Verification items for the finished model (mm, model axes). Face numbers are marked on the shaded views. A direction names the side the tool comes from. Give positions to 0.01 mm unless a question says otherwise; leave off trailing zeros. Order: outer loops, then holes, each group sorted by start corner. A loop starts at its lowest first (then second) coordinate and runs counter-clockwise, first axis right, second up. Notation, with made-up numbers: (63.5, 11.25) - (104.5, 11.25) arc R14 ccw to (104.5, 38.25) - close; hole circle Ø1 at (-17.5, 76). An arc over 180 degrees is marked (long way). Answer as a JSON object with one key per item and string values.
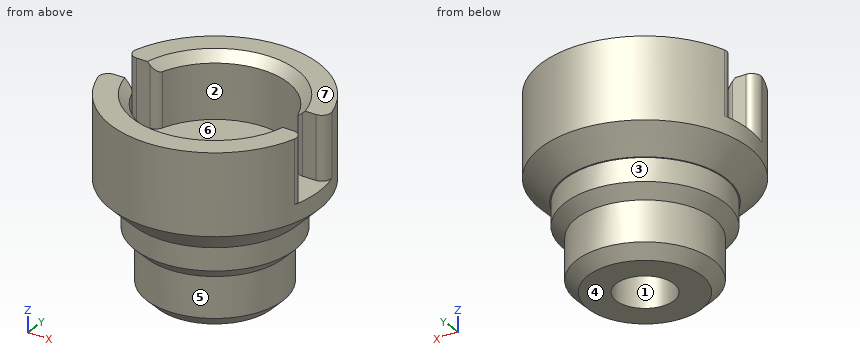
```python
from build123d import *

# Parameters (mm, degrees)
SKETCH1_R           = 2.95
SKETCH1_R_2         = 1.25
BOSS_EXTRUDE1_DEPTH = 3.75
SKETCH2_R           = 4.5
SKETCH2_R_2         = 1.25
BOSS_EXTRUDE2_DEPTH = 4.5
SKETCH3_R           = 3.15
CUT_EXTRUDE1_DEPTH  = 2.75
CHAMFER1_SIZE       = 0.4
CHAMFER2_SIZE       = 0.5
BOSS_EXTRUDE3_START = 1.5
SKETCH4_R           = 3.45
SKETCH4_R_2         = 1.25
BOSS_EXTRUDE3_DEPTH = 1.5
CHAMFER3_SIZE       = 1
CHAMFER6_SIZE       = 0.5
CUT_EXTRUDE2_REACH  = 12.419
SKETCH5_W           = 12.167806538
SKETCH5_H           = 1.5
FILLET1_R           = 0.4


with BuildPart() as part:
    # Sketch1 → Boss-Extrude1 (new body)
    with BuildSketch(Plane.XY):
        Circle(SKETCH1_R)
        Circle(SKETCH1_R_2, mode=Mode.SUBTRACT)
    extrude(amount=BOSS_EXTRUDE1_DEPTH)

    # Sketch2 → Boss-Extrude2 (add)
    with BuildSketch(Plane.XY.offset(3.75)):
        Circle(SKETCH2_R)
        Circle(SKETCH2_R_2, mode=Mode.SUBTRACT)
    extrude(amount=BOSS_EXTRUDE2_DEPTH)

    # Sketch3 → Cut-Extrude1 (cut)
    with BuildSketch(Plane.XY.offset(8.25)):
        Circle(SKETCH3_R)
    extrude(amount=-CUT_EXTRUDE1_DEPTH, mode=Mode.SUBTRACT)

    # Chamfer1
    chamfer1_edges = [part.edges().sort_by_distance(p)[0] for p in [
        (-3.15, 0, 8.25),
    ]]
    chamfer(chamfer1_edges, length=CHAMFER1_SIZE)

    # Chamfer2
    chamfer2_edges = [part.edges().sort_by_distance(p)[0] for p in [
        (-2.95, 0, 0),
    ]]
    chamfer(chamfer2_edges, length=CHAMFER2_SIZE)

    # Sketch4 → Boss-Extrude3 (add)
    with BuildSketch(Plane(origin=(0, 0, 3.75), x_dir=(-1, 0, 0), z_dir=(0, 0, -1)).offset(BOSS_EXTRUDE3_START)):
        with Locations(Location((0, 0, 0), (0, 0, 180))):
            Circle(SKETCH4_R)
        with Locations(Location((0, 0, 0), (0, 0, 180))):
            Circle(SKETCH4_R_2, mode=Mode.SUBTRACT)
    extrude(amount=-BOSS_EXTRUDE3_DEPTH)

    # Chamfer3
    chamfer3_edges = [part.edges().sort_by_distance(p)[0] for p in [
        (-4.5, 0, 3.75),
    ]]
    chamfer(chamfer3_edges, length=CHAMFER3_SIZE)

    # Chamfer6
    chamfer6_edges = [part.edges().sort_by_distance(p)[0] for p in [
        (-3.45, 0, 2.25),
    ]]
    chamfer(chamfer6_edges, length=CHAMFER6_SIZE - 0.0001)  # a hair under: the kernel refuses the full size

    # Cut-Extrude2: up to this face of the body (flat: up to its plane)
    cut_extrude2_end = Plane(part.part.faces().sort_by_distance((-3.060904546, 0, 5.5))[0])
    # Sketch5 → Cut-Extrude2 (cut, up to the picked face)
    with BuildSketch(Plane.XY.offset(8.25), mode=Mode.PRIVATE) as cut_extrude2_sk1:
        Rectangle(SKETCH5_W, SKETCH5_H)
    cut_extrude2_tool1 = split(extrude(cut_extrude2_sk1.sketch, amount=-CUT_EXTRUDE2_REACH, mode=Mode.PRIVATE), bisect_by=cut_extrude2_end, keep=Keep.BOTH, mode=Mode.PRIVATE)
    add(cut_extrude2_tool1.solids().sort_by(Axis((0, 0, 8.25), (0, 0, -1)))[0], mode=Mode.SUBTRACT)

    # Fillet1
    fillet1_edges = [part.edges().sort_by_distance(p)[0] for p in [
        (3.059411708, -0.75, 6.675),
        (-3.059411708, -0.75, 6.675),
        (4.437059837, -0.75, 6.875),
        (-4.437059837, -0.75, 6.875),
        (-3.059411708, 0.75, 6.675),
        (3.059411708, 0.75, 6.675),
        (-4.437059837, 0.75, 6.875),
        (4.437059837, 0.75, 6.875),
    ]]
    fillet(fillet1_edges, radius=FILLET1_R)


solid = part.part
```
(1) Section check C-C (z = 6.5). Record the cut outline in (x, y).
Computed values:
{"outline": "(-4.32, -1.26) arc R4.5 ccw to (4.32, -1.26) arc R0.4 ccw to (3.94, -0.75) - (3.36, -0.75) arc R0.4 ccw to (2.98, -1.02) arc R3.15 cw to (-2.98, -1.02) arc R0.4 ccw to (-3.36, -0.75) - (-3.94, -0.75) arc R0.4 ccw to start; (-4.32, 1.26) arc R0.4 ccw to (-3.94, 0.75) - (-3.36, 0.75) arc R0.4 ccw to (-2.98, 1.02) arc R3.15 cw to (2.98, 1.02) arc R0.4 ccw to (3.36, 0.75) - (3.94, 0.75) arc R0.4 ccw to (4.32, 1.26) arc R4.5 ccw to start"}
(2) Gauge pin test, flat ends, axial feed: pin 1 Ø0.6 at (x, z) = (3.5, 6.5) entering from +Y; pin 2 Ø0.6 at (x, z) = (-3.5, 7) entering from -Y; pin 3 Ø0.5 at (x, z) = (3.5, 7) entering from -Y. Record the tip position at first contact, or that the pin passes through.
Computed values:
{"pin 1": "stops at y = 3.16", "pin 2": "stops at y = -3.16", "pin 3": "stops at y = -3.11"}
(3) Release check for a two-part mould opening along Y. For the marked faces 1, 2, 3 and 4 record: pulls with the +Y half, pulls with the -Y half, needs draft (parallel to the pull), parting line crosses it, or undercut.
Computed values:
{"face 1": "undercut", "face 2": "undercut", "face 3": "parting line crosses it", "face 4": "needs draft"}
(4) Access from +Z, -Z, +X, -X, +Y, -Y to the whole of each face (thin tool, end or side, straight path). Record for the marked faces 5, 6 and 7.
Computed values:
{"face 5": "-Z", "face 6": "+Z", "face 7": "+Z, +X, -X, +Y, -Y"}
(5) Section check D-D (z = 4.25). Record the cut outline in (x, y).
Computed values:
{"outline": "circle Ø8 at (0, 0); hole circle Ø2.5 at (0, 0)"}
(6) Material ranges on line 1 along X through (y, z) = (0, 1.3); line 2 along Z through (x, y) = (-0.75, 1.75), recorded low to high. Write a range as [from, to].
Computed values:
{"line 1": "x = [-2.95, -1.25], [1.25, 2.95]", "line 2": "z = [0, 5.5]"}
